Can you work these out from the model? Positions are in its coordinate system, mm. A direction names the side the tool comes from. Give positions to 0.01 mm unless a question says otherwise; leave off trailing zeros. Write each loop counter-clockwise with the first axis right and the second up, starting at its lowest first coordinate (ties: lowest second). Pieces come first, ordered by that corner, then holes. Notation, with made-up numbers: M -4,31 L 17,31 A24 cw 17,44 Z; hole C 14.5,59.5 d3. An arc over 180 degrees is marked long. Use CSV: the item, a comma, the result in double quotes. Start each with the question number.
from build123d import *

# Parameters (mm, degrees)
F0_W     = 32
F0_H     = 45
F1_DEPTH = 1
F3_DEPTH = 3.5
F4_R     = 3.49999


# Not quite as in the source:
# - a fillet or chamfer is up to 0.001 mm smaller than in the source, because OpenCascade refuses the exact size


with BuildPart() as f1:
    # F0 (on Front) → F1 (new body)
    with BuildSketch(Plane.XZ):
        with BuildLine():
            Line((16, 22.5), (16, -22.5))
            ThreePointArc((16, -22.5), (38.5, 0), (16, 22.5))
        make_face()
        Rectangle(F0_W, F0_H)
        with BuildLine():
            ThreePointArc((-16, 22.5), (-38.5, 0), (-16, -22.5))
            Line((-16, -22.5), (-16, 22.5))
        make_face()
    extrude(amount=F1_DEPTH)

    # F2 (on face) → F3 (join)
    with BuildSketch(Plane.XZ.offset(1)):
        with BuildLine():
            ThreePointArc((16, -19), (35, 0), (16, 19))
            Line((16, 19), (-16, 19))
            ThreePointArc((-16, 19), (-35, 0), (-16, -19))
            Line((-16, -19), (16, -19))
        make_face()
        with BuildLine():
            ThreePointArc((-16, -12), (-28, 0), (-16, 12))
            Line((-16, 12), (16, 12))
            ThreePointArc((16, 12), (28, 0), (16, -12))
            Line((16, -12), (-16, -12))
        make_face(mode=Mode.SUBTRACT)
    extrude(amount=F3_DEPTH)

    # F4 (radius 3.5 in the source; OpenCascade refuses exactly that, so slightly less here)
    f4_edges = [f1.edges().sort_by_distance(p)[0] for p in [
        (0, -4.5, 19),
        (0, -4.5, 12),
    ]]
    fillet(f4_edges, radius=F4_R)


solid = f1.part
(1) I want a section at B-B (y = -3.35). Write out the boundary of the cut face in (x, z), and give its area (3 significant figures).
(2) Please list where these lines run through material, in increasing order: L1, parallel to Z at x = 7.5, y = -1.05; L2, parallel to Y at x = 21, z = 3.5; L3, parallel to Z at x = -13, y = -1.6. Write a range as [from, to].
(3) Thinking about a two-plate mould opening in X: for faces 3 (the face through (38.495, -0.493, -0.495)), 4 (the face through (0.22, -3.5, 13.05)), 5 (the face through (-0.22, -3.45, 18)), which applies, released by +X, released by -X, zero draft, split by the parting line, or undercut?
(4) Will these pins go through, and if not, where does the flat tip stop? pin 1 Ø1 at (y, z) = (-3.5, 10) entering from +X; pin 2 Ø19 at (x, z) = (-5.5, 1.5) entering from -Y.
(5) Which directions (+Z, -Z, +X, -X, +Y, -Y) give clear straight access to the entire face, cutting with the end or side of a thin tool? Please do faces 1 (the face through (0, -1, -20)), 2 (the face through (-1, 0, 0)).
Geometry results:
1,outline,"M -16,-18.09 L 16,-18.09 A18.09 ccw 16,18.09 L -16,18.09 A18.09 ccw Z; hole M -16,-12.91 L 16,-12.91 A12.91 ccw 16,12.91 L -16,12.91 A12.91 ccw Z"
1,area,"837 mm2"
2,L1,"z = [-19, -12], [12, 19]"
2,L2,"y = [-1, 0]"
2,L3,"z = [-18.95, -12.05], [12.05, 18.95]"
3,face 3,"released by +X"
3,face 4,"undercut"
3,face 5,"zero draft"
4,pin 1,"stops at x = 31.52"
4,pin 2,"stops at y = -1"
5,face 1,"-Y"
5,face 2,"+Z, -Z, +X, -X, +Y"
